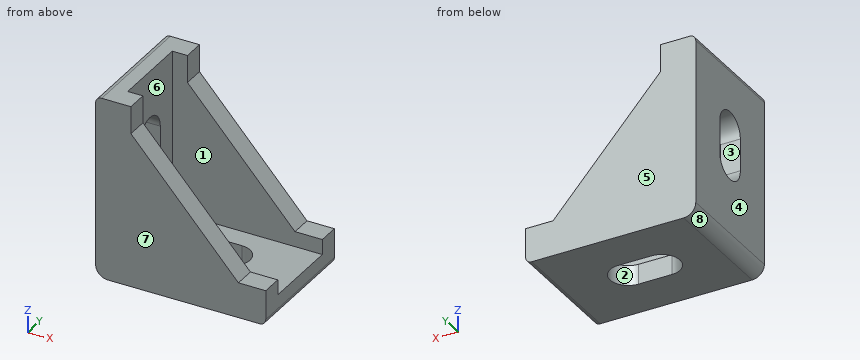
```python
from build123d import *

# Parameters (mm, degrees)
SKETCH1_W           = 28
SKETCH1_H           = 20
BOSS_EXTRUDE1_DEPTH = 3.3
SKETCH2_W           = 3.3
SKETCH2_H           = 20
BOSS_EXTRUDE2_DEPTH = 26.7
CUT_EXTRUDE1_DEPTH  = 44.704576419
BOSS_EXTRUDE3_DEPTH = 3.5
BOSS_EXTRUDE4_DEPTH = 3.5
FILLET1_R           = 2
FILLET2_R           = 1
FILLET3_R           = 1


with BuildPart() as part:
    # Sketch1 → Boss-Extrude1 (new body)
    with BuildSketch(Plane.XY):
        with Locations((14, 10)):
            Rectangle(SKETCH1_W, SKETCH1_H)
        with BuildLine():
            Line((11.25, 13), (16.75, 13))
            ThreePointArc((16.75, 13), (19.75, 10), (16.75, 7))
            Line((16.75, 7), (11.25, 7))
            ThreePointArc((11.25, 7), (8.25, 10), (11.25, 13))
        make_face(mode=Mode.SUBTRACT)
    extrude(amount=BOSS_EXTRUDE1_DEPTH)

    # Sketch2 → Boss-Extrude2 (add)
    with BuildSketch(Plane.XY.offset(3.3)):
        with Locations((1.65, 10)):
            Rectangle(SKETCH2_W, SKETCH2_H)
    extrude(amount=BOSS_EXTRUDE2_DEPTH)

    # Sketch3 → Cut-Extrude1 (cut, through all)
    with BuildSketch(Plane(origin=(3.3, 0, 0), x_dir=(0, 0, -1), z_dir=(1, 0, 0))):
        with BuildLine():
            Line((-19.3, 13), (-14, 13))
            ThreePointArc((-14, 13), (-11, 10), (-14, 7))
            Line((-14, 7), (-19.3, 7))
            ThreePointArc((-19.3, 7), (-22.3, 10), (-19.3, 13))
        make_face()
    extrude(amount=-CUT_EXTRUDE1_DEPTH, mode=Mode.SUBTRACT)

    # Sketch4 → Boss-Extrude3 (add)
    with BuildSketch(Plane.XZ):
        Polygon((3.3, 30), (5.8, 30), (5.8, 25.5), (23.5, 5.8), (28, 5.8), (28, 3.3), (3.3, 3.3), align=None)
    extrude(amount=-BOSS_EXTRUDE3_DEPTH)

    # Sketch5 → Boss-Extrude4 (add)
    with BuildSketch(Plane(origin=(0, 20, 0), x_dir=(1, 0, 0), z_dir=(0, 1, 0))):
        Polygon((28, -3.3), (28, -5.8), (23.5, -5.8), (5.8, -25.5), (5.8, -30), (3.3, -30), (3.3, -3.3), align=None)
    extrude(amount=-BOSS_EXTRUDE4_DEPTH)

    # Fillet1
    fillet1_edges = [part.edges().sort_by_distance(p)[0] for p in [
        (0, 10, 0),
    ]]
    fillet(fillet1_edges, radius=FILLET1_R)

    # Fillet2
    fillet2_edges = [part.edges().sort_by_distance(p)[0] for p in [
        (0, 10, 30),
    ]]
    fillet(fillet2_edges, radius=FILLET2_R)

    # Fillet3
    fillet3_edges = [part.edges().sort_by_distance(p)[0] for p in [
        (28, 10, 0),
    ]]
    fillet(fillet3_edges, radius=FILLET3_R)


solid = part.part
```
Can you work these out from the model? Positions are in its coordinate system, mm. Face numbers are marked on the shaded views. A direction names the side the tool comes from. Round coordinates to 2 decimals unless told otherwise and drop trailing zeros. Loops run counter-clockwise (first coordinate to the right, second up) from the corner with the lowest first, then second, coordinate; pieces in that order, holes last. Notation, with made-up numbers: M 21.5,47 L 71.5,47 A23 ccw 71.5,57 Z; hole C 46,-7.5 d9. An arc over 180 degrees is marked long. Answer as a JSON object with one key per item and string values. Group by question number.
Q1. Imagine slicing it at A-A, the plane y = 10. Please give me the cut outline in (x, z).
Q2. On a 3-axis mill with a long thin cutter (end or side, diameter ignored), from which of +Z, -Z, +X, -X, +Y, -Y can I reach the whole of each face in a straight line? I mean the marked faces 1, 2, 3 and 4. Say none if no direction works.
Q3. Imagine slicing it at C-C, the plane x = 15.5. Please give me the cut outline in (y, z), then the cut area to 3 significant figures.
Q4. Will these pins go through, and if not, where does the flat tip stop? pin 1 (3 mm diameter, centred on y = 2, z = 28.5, fed in from +X); pin 2 (1.8 mm diameter, centred on x = 26, y = 19, fed in from +Z); pin 3 (1.5 mm diameter, centred on y = 10, z = 10, fed in from +X); pin 4 (5 mm diameter, centred on x = 15.5, z = 17.5, fed in from -Y).
Q5. We'd pull the mould along Y, two halves only. Please class the marked faces 5, 6, 7 and 8: +Y half, -Y half, draft (parallel to the pull), parting line (faces both ways), or undercut.
Q6. Please list where these lines run through material, in increasing order: L1, parallel to Y at x = 13, z = 3.25; L2, parallel to Y at x = 6, z = 9.25; L3, parallel to Z at x = 26.25, y = 17.
Q7. Imagine slicing it at B-B, the plane z = 12. Please give me the cut outline in (x, y), then the cut area to 3 significant figures.
Q8. Imagine slicing it at D-D, the plane y = 4.5. Please give me the cut outline in (x, z).
Findings:
{
 "1": {"outline": "M 0,2 A2 ccw 2,0 L 8.25,0 L 8.25,3.3 L 3.3,3.3 L 3.3,11 L 0,11 Z; M 0,22.3 L 3.3,22.3 L 3.3,30 L 1,30 A1 ccw 0,29 Z; M 19.75,0 L 27,0 A1 ccw 28,1 L 28,3.3 L 19.75,3.3 Z"},
 "2": {"face 1": "+Z, +X", "face 2": "+Z, -Z", "face 3": "+X, -X", "face 4": "+Z, -Z, -X, +Y, -Y"},
 "3": {"outline": "M 0,0 L 7,0 L 7,3.3 L 3.5,3.3 L 3.5,14.7 L 0,14.7 Z; M 13,0 L 20,0 L 20,14.7 L 16.5,14.7 L 16.5,3.3 L 13,3.3 Z", "area": "126 mm2"},
 "4": {"pin 1": "stops at x = 5.8", "pin 2": "stops at z = 5.8", "pin 3": "stops at x = 3.3", "pin 4": "stops at y = 0"},
 "5": {"face 5": "+Y half", "face 6": "undercut", "face 7": "-Y half", "face 8": "draft"},
 "6": {"L1": "y = 0 to 7, 13 to 20", "L2": "y = 0 to 3.5, 16.5 to 20", "L3": "z = 0 to 5.8"},
 "7": {"outline": "M 0,0 L 17.93,0 L 17.93,3.5 L 3.3,3.5 L 3.3,7.76 L 0,7.76 Z; M 0,12.24 L 3.3,12.24 L 3.3,16.5 L 17.93,16.5 L 17.93,20 L 0,20 Z", "area": "154 mm2"},
 "8": {"outline": "M 0,2 A2 ccw 2,0 L 27,0 A1 ccw 28,1 L 28,3.3 L 3.3,3.3 L 3.3,30 L 1,30 A1 ccw 0,29 Z"}
}
